Source: CAD feature listing. Evaluate the final solid. Frame: model axes, mm. Face numbers are marked on the shaded views. Give positions to 0.01 mm unless a question says otherwise; leave off trailing zeros. Write each loop counter-clockwise with the first axis right and the second up, starting at its lowest first coordinate (ties: lowest second). Pieces come first, ordered by that corner, then holes. Notation, with made-up numbers: (11, -20) - (19, -20) arc R27 cw to (19, -2) - close; hole circle Ø4 at (62, -22). An arc over 180 degrees is marked (long way). One line per question, with ' | ' between items. Start each with the question number.
(1) Ray query, line 1 (Y direction, x = 1.7, z = 0); line 2 (Y direction, x = 3, z = -1.4); line 3 (Y direction, x = 1.9, z = -0.2). Return the intervals inside material, ascending. Write a range as [from, to].
(2) Section B-B, the plane x = 3. Return loops of the section in (y, z), plus the area to 3 significant figures.
(3) Section A-A, the plane z = 0. Return loops of the section in (x, y), plus the area to 3 significant figures.
(4) Pin query (flat end, axial travel): pin 1 (2 mm diameter, centred on y = 8, z = 0, fed in from +X) (1 decimal). Return the tip coordinate at first contact, or that it passes through.
(5) Section D-D, the plane x = 0.8. Return loops of the section in (y, z), plus the area to 3 significant figures.
(6) Draft query along Y for the marked faces 1, 2, 3 and 4. Return one class per face: +Y half, -Y half, draft (parallel to the pull), parting line (faces both ways), or undercut.
(7) Section C-C, the plane y = -8. Return loops of the section in (x, z), plus the area to 3 significant figures.
```python
from build123d import *

# Parameters (mm, degrees)
SKETCH_1_W          = 6
SKETCH_1_H          = 22
SKETCH_1_R          = 1.25
EXTRUDE_1_DEPTH     = 6
SKETCH_2_R          = 1.25
CUT_EXTRUDE_1_DEPTH = 7


with BuildPart() as part:
    # 草图1 → 凸台-拉伸1 (new body)
    with BuildSketch(Plane(origin=(0, 0, 0), x_dir=(0, 0, -1), z_dir=(1, 0, 0))):
        Rectangle(SKETCH_1_W, SKETCH_1_H)
        with Locations((0, 8)):
            Circle(SKETCH_1_R, mode=Mode.SUBTRACT)
        with Locations((0, -8)):
            Circle(SKETCH_1_R, mode=Mode.SUBTRACT)
    extrude(amount=EXTRUDE_1_DEPTH)

    # 草图2 → 切除-拉伸1 (cut, through all)
    with BuildSketch(Plane.XY.offset(3)):
        with Locations((3, 0)):
            Circle(SKETCH_2_R)
    extrude(amount=-CUT_EXTRUDE_1_DEPTH, mode=Mode.SUBTRACT)


solid = part.part
```
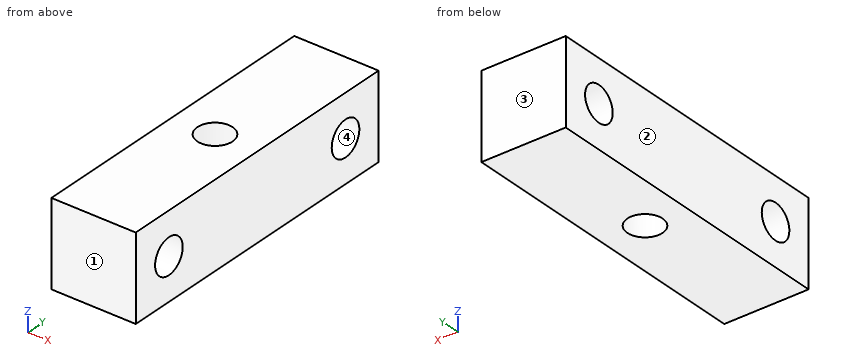
Check sheet entries:
1) line 1: [-11, -9.25], [-6.75, 6.75], [9.25, 11] | line 2: [-11, -1.25], [1.25, 11] | line 3: [-11, -9.23], [-6.77, -0.59], [0.59, 6.77], [9.23, 11]
2) outline: (-11, -3) - (-1.25, -3) - (-1.25, 3) - (-11, 3) - close; (1.25, -3) - (11, -3) - (11, 3) - (1.25, 3) - close; hole circle Ø2.5 at (-8, 0); hole circle Ø2.5 at (8, 0) | area: 107 mm²
3) outline: (0, -11) - (6, -11) - (6, -9.25) - (0, -9.25) - close; (0, -6.75) - (6, -6.75) - (6, 6.75) - (0, 6.75) - close; (0, 9.25) - (6, 9.25) - (6, 11) - (0, 11) - close; hole circle Ø2.5 at (3, 0) | area: 97.1 mm²
4) pin 1: through
5) outline: (-11, -3) - (11, -3) - (11, 3) - (-11, 3) - close; hole circle Ø2.5 at (-8, 0); hole circle Ø2.5 at (8, 0) | area: 122 mm²
6) face 1: -Y half | face 2: draft | face 3: +Y half | face 4: undercut
7) outline: (0, -3) - (6, -3) - (6, -1.25) - (0, -1.25) - close; (0, 1.25) - (6, 1.25) - (6, 3) - (0, 3) - close | area: 21.0 mm²
